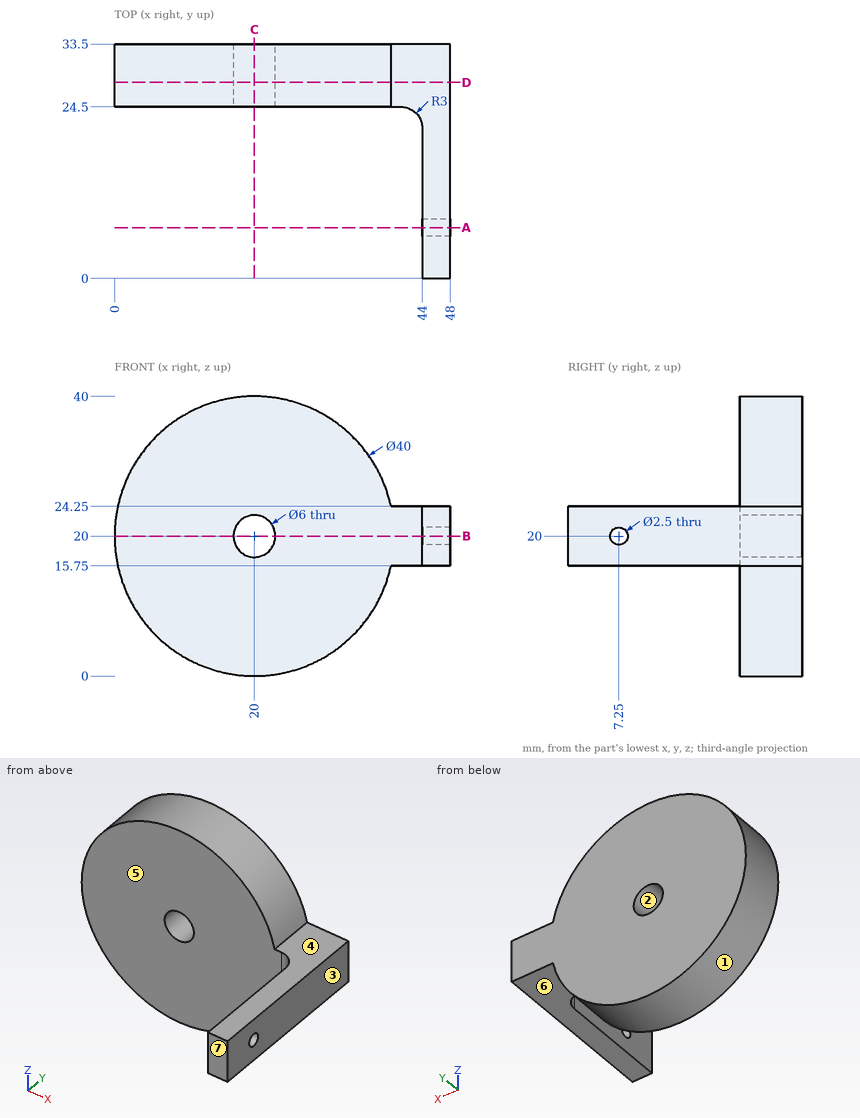
Answer from the drawing. Dimensions are ordinates in mm from the lowest x, y and z of the part. A direction names the side the tool comes from. Coordinates: 2 decimals unless noted, no trailing zeros. Order: outer loops, then holes, each group sorted by start corner. A loop starts at its lowest first (then second) coordinate and runs counter-clockwise, first axis right, second up. Notation, with made-up numbers: (1.5, 44) -> (20.5, 44) arc R20 ccw to (20.5, 62) -> close; hole circle Ø7 at (57, 27). An arc over 180 degrees is marked (long way). Answer as a JSON object with one key per item and string values.
1) Each of these flat-tipped pins is pushed along its axis until it touches: pin 1 (12 mm diameter, centred on y = 18, z = 10, fed in from -X); pin 2 (9.5 mm diameter, centred on x = 45, y = 23.5, fed in from +Z); pin 3 (5 mm diameter, centred on x = 42, y = 18, fed in from +Z). Where does it stop, or does it pass through?
Model answer:
{"pin 1": "stops at x = 44", "pin 2": "stops at z = 24.25", "pin 3": "stops at z = 24.25"}
2) A tool of negligible diameter and unlimited length cuts with its end or side. For the marked faces 4, 5, 6 and 7, from which of +Z, -Z, +X, -X, +Y, -Y can it reach the whole face along a straight path? Write none if from no direction.
Model answer:
{"face 4": "+Z, +X, +Y, -Y", "face 5": "+Z, -Z, -X, -Y", "face 6": "-Z, +X, +Y, -Y", "face 7": "+Z, -Z, +X, -X, -Y"}
3) A cutting plane is placed at B-B, the plane z = 20. Determine the outline of the cut face in (x, y).
Model answer:
{"outline": "(0, 24.5) -> (17, 24.5) -> (17, 33.5) -> (0, 33.5) -> close; (23, 24.5) -> (41, 24.5) arc R3 cw to (44, 21.5) -> (44, 8.5) -> (48, 8.5) -> (48, 33.5) -> (23, 33.5) -> close; (44, 0) -> (48, 0) -> (48, 6) -> (44, 6) -> close"}
4) Consider line 1 along Y through (x, z) = (13, 3); line 2 along X through (y, z) = (17.5, 20); line 3 along Z through (x, y) = (20, 31). Determine where each line is inside the solid, lowest interval first. Write a range as from..to.
Model answer:
{"line 1": "y = 24.5..33.5", "line 2": "x = 44..48", "line 3": "z = 0..17, 23..40"}
5) A cutting plane is placed at D-D, the plane y = 28. Determine the outline of the cut face in (x, z), plus the area to 3 significant figures.
Model answer:
{"outline": "(39.54, 15.75) -> (48, 15.75) -> (48, 24.25) -> (39.54, 24.25) arc R20 ccw (long way) to start; hole circle Ø6 at (20, 20)", "area": "1,300 mm²"}
6) A cutting plane is placed at C-C, the plane x = 20. Determine the outline of the cut face in (y, z), plus the area to 3 significant figures.
Model answer:
{"outline": "(24.5, 0) -> (33.5, 0) -> (33.5, 17) -> (24.5, 17) -> close; (24.5, 23) -> (33.5, 23) -> (33.5, 40) -> (24.5, 40) -> close", "area": "306 mm²"}
7) A cutting plane is placed at A-A, the plane y = 7.25. Determine the outline of the cut face in (x, z), plus the area to 3 significant figures.
Model answer:
{"outline": "(44, 15.75) -> (48, 15.75) -> (48, 18.75) -> (44, 18.75) -> close; (44, 21.25) -> (48, 21.25) -> (48, 24.25) -> (44, 24.25) -> close", "area": "24.0 mm²"}
8) The mould has two halves that part along Z. Classify the marked faces 1, 2 and 3: released by +Z, released by -Z, zero draft, split by the parting line, or undercut.
Model answer:
{"face 1": "split by the parting line", "face 2": "undercut", "face 3": "zero draft"}
